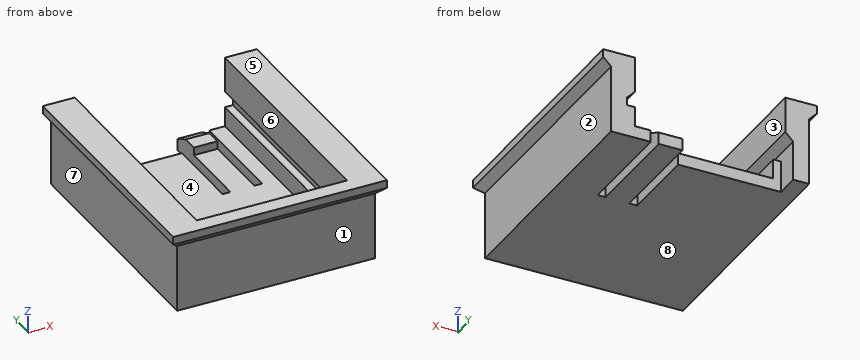
from build123d import *

# Parameters (mm, degrees)
SKETCH1_W               = 25
SKETCH1_H               = 10.5
BOSS_EXTRUDE1_DEPTH     = 31
CUT_EXTRUDE1_DEPTH      = 30
SKETCH8_W               = 3
SKETCH8_H               = 2
BOSS_EXTRUDE4_DEPTH     = 1
CHAMFER1_SIZE2          = 1
CHAMFER1_SIZE           = 2
CUT_EXTRUDE_THIN1_DEPTH = 35.615747861
CUT_EXTRUDE5_REACH      = 37.036
SKETCH10_W              = 13
SKETCH10_H              = 3
EXTRUDE_THIN1_DEPTH     = 1
CHAMFER2_SIZE           = 1
CHAMFER3_SIZE           = 1


with BuildPart() as part:
    # Sketch1 → Boss-Extrude1 (new body)
    with BuildSketch(Plane(origin=(0, 0, 0), x_dir=(1, 0, 0), z_dir=(0, 1, 0))):
        Rectangle(SKETCH1_W, SKETCH1_H)
    extrude(amount=BOSS_EXTRUDE1_DEPTH)

    # Sketch2 → Cut-Extrude1 (cut)
    with BuildSketch(Plane(origin=(0, 31, 0), x_dir=(1, 0, 0), z_dir=(0, 1, 0))):
        Polygon((-9.5, 3.75), (9.5, 3.75), (9.5, 1.25), (10.5, 1.25), (10.5, -0.75), (9.5, -0.75), (9.5, -5.25), (-9.5, -5.25), (-9.5, -0.75), (-10.5, -0.75), (-10.5, 1.25), (-9.5, 1.25), align=None)
    extrude(amount=-CUT_EXTRUDE1_DEPTH, mode=Mode.SUBTRACT)

    # Sketch8 → Boss-Extrude4 (add)
    with BuildSketch(Plane.XY.offset(-3.75)):
        with Locations((5, 28)):
            Rectangle(SKETCH8_W, SKETCH8_H)
    extrude(amount=BOSS_EXTRUDE4_DEPTH)

    # Chamfer1
    chamfer1_edges = [part.edges().sort_by_distance(p)[0] for p in [
        (5, 29, -3.75),
    ]]
    chamfer1_side = [part.faces().sort_by_distance(p)[0] for p in [
        (5, 29.02, -3.75),
    ]]
    chamfer(chamfer1_edges, length=CHAMFER1_SIZE - 0.0001, length2=CHAMFER1_SIZE2 - 0.0001, reference=chamfer1_side[0])  # a hair under: the kernel refuses the full size

    # Sketch9 → Cut-Extrude-Thin1 (cut, through all)
    with BuildSketch(Plane.XY.offset(-3.75)):
        Polygon((6.5, 18), (6.5, 31), (3.5, 31), (3.5, 18), (2.5, 18), (2.5, 32), (7.5, 32), (7.5, 18), align=None)
    extrude(amount=-CUT_EXTRUDE_THIN1_DEPTH, mode=Mode.SUBTRACT)

    # Sketch10 → Cut-Extrude5 (cut, up to next)
    with BuildSketch(Plane(origin=(0, 0, -5.25), x_dir=(-1, 0, 0), z_dir=(0, 0, -1)), mode=Mode.PRIVATE) as cut_extrude5_sk1:
        with Locations((4, 29.5)):
            Rectangle(SKETCH10_W, SKETCH10_H)
    cut_extrude5_tool1 = extrude(cut_extrude5_sk1.sketch, amount=-CUT_EXTRUDE5_REACH, mode=Mode.PRIVATE) & part.part
    add(cut_extrude5_tool1.solids().sort_by_distance((-4, 29.5, -5.25))[0], mode=Mode.SUBTRACT)

    # Sketch11 → Extrude-Thin1 (add)
    with BuildSketch(Plane.XY.offset(5.25)):
        Polygon((12.5, 31), (12.5, 0), (-12.5, 0), (-12.5, 31), (-13.5, 31), (-13.5, -1), (13.5, -1), (13.5, 31), align=None)
    extrude(amount=-EXTRUDE_THIN1_DEPTH)

    # Chamfer2
    chamfer2_edges = [part.edges().sort_by_distance(p)[0] for p in [
        (-12.5, 15.5, 4.25),
        (0, 0, 4.25),
        (12.5, 15.5, 4.25),
    ]]
    chamfer(chamfer2_edges, length=CHAMFER2_SIZE - 0.0001)  # a hair under: the kernel refuses the full size

    # Chamfer3
    chamfer3_edges = [part.edges().sort_by_distance(p)[0] for p in [
        (-10.5, 16, 0.75),
        (10.5, 16, 0.75),
    ]]
    chamfer(chamfer3_edges, length=CHAMFER3_SIZE - 0.0001)  # a hair under: the kernel refuses the full size


solid = part.part
Geometry: final body of the model. Coordinates: model frame, mm. Face numbers are marked on the shaded views. A direction names the side the tool comes from. Coordinates: 2 decimals unless noted, no trailing zeros. Loops run counter-clockwise (first coordinate to the right, second up) from the corner with the lowest first, then second, coordinate; pieces in that order, holes last. Notation, with made-up numbers: (-24.5, 20.5) - (14.5, 20.5) arc R10 cw to (14.5, 33.5) - close; hole circle Ø4 at (48.25, -6). An arc over 180 degrees is marked (long way). Put each result on its own line as item: value. Start each with the question number.
Q1. Cut plane A-A, the plane y = 20. Give the number of separate pieces and of enclosed holes in the cut face, and give its area (3 significant figures).
Q2. Set-up query: the marked faces 1, 2, 3, 4 and 5. Return all of +Z, -Z, +X, -X, +Y, -Y with unobstructed straight access to the full face (end or side cutting, diameter ignored); none if empty.
Q3. Cut plane B-B, the plane z = -3.25. Return loops of the section in (x, y), and give its area (3 significant figures).
Q4. Pin query (flat end, axial travel): pin 1 Ø9.5 at (x, y) = (3.5, 11) entering from +Z; pin 2 Ø6 at (y, z) = (7.5, 3.5) entering from +X; pin 3 Ø0.8 at (x, z) = (7, -4) entering from +Y; pin 4 Ø2 at (y, z) = (11.5, -3) entering from -X. Return the tip coordinate at first contact, or that it passes through.
Q5. Pull-direction query (X, two-part tool) for the marked faces 6, 7 and 8; classes: released by +X, released by -X, zero draft, split by the parting line, or undercut.
Q6. Line query: line 1 (X direction, y = 3, z = -2.25); line 2 (X direction, y = 7.5, z = -0.25); line 3 (Z direction, x = 7.5, y = 4). Output: solid intervals per line, ascending.
Filled sheet:
1. separate pieces: 3
1. enclosed holes: 0
1. area: 88.5 mm²
2. face 1: -Z, +X, -X, -Y
2. face 2: -Z, +X, +Y, -Y
2. face 3: +Z, +Y
2. face 4: +Z
2. face 5: +Z, +X, -X, +Y, -Y
3. outline: (-12.5, 0) - (12.5, 0) - (12.5, 31) - (9.5, 31) - (9.5, 1) - (-9.5, 1) - (-9.5, 28) - (-10.5, 28) - (-10.5, 31) - (-12.5, 31) - close; (3.5, 27) - (6.5, 27) - (6.5, 30) - (3.5, 30) - close
3. area: 211 mm²
4. pin 1: z = -3.75
4. pin 2: x = 13.5
4. pin 3: y = 18
4. pin 4: x = -12.5
5. face 6: undercut
5. face 7: released by -X
5. face 8: zero draft
6. line 1: -12.5 to -9.5, 9.5 to 12.5
6. line 2: -12.5 to -10.5, 10.5 to 12.5
6. line 3: -5.25 to -3.75
